Study the drawing (mm; zero at the part's minimum x, y, z) and answer. A direction names the side the tool comes from. Coordinates: 2 decimals unless noted, no trailing zeros. Write each loop counter-clockwise with the first axis right and the second up, starting at its lowest first coordinate (ties: lowest second). Pieces come first, ordered by that corner, then holes. Notation, with made-up numbers: (-16, -21) -> (27, -21) arc R15 ccw to (27, -17) -> close; hole circle Ø1 at (63.25, -21.75). An arc over 180 degrees is marked (long way). Write each question's results on one line, items separated by ' | '. Start each with the question number.
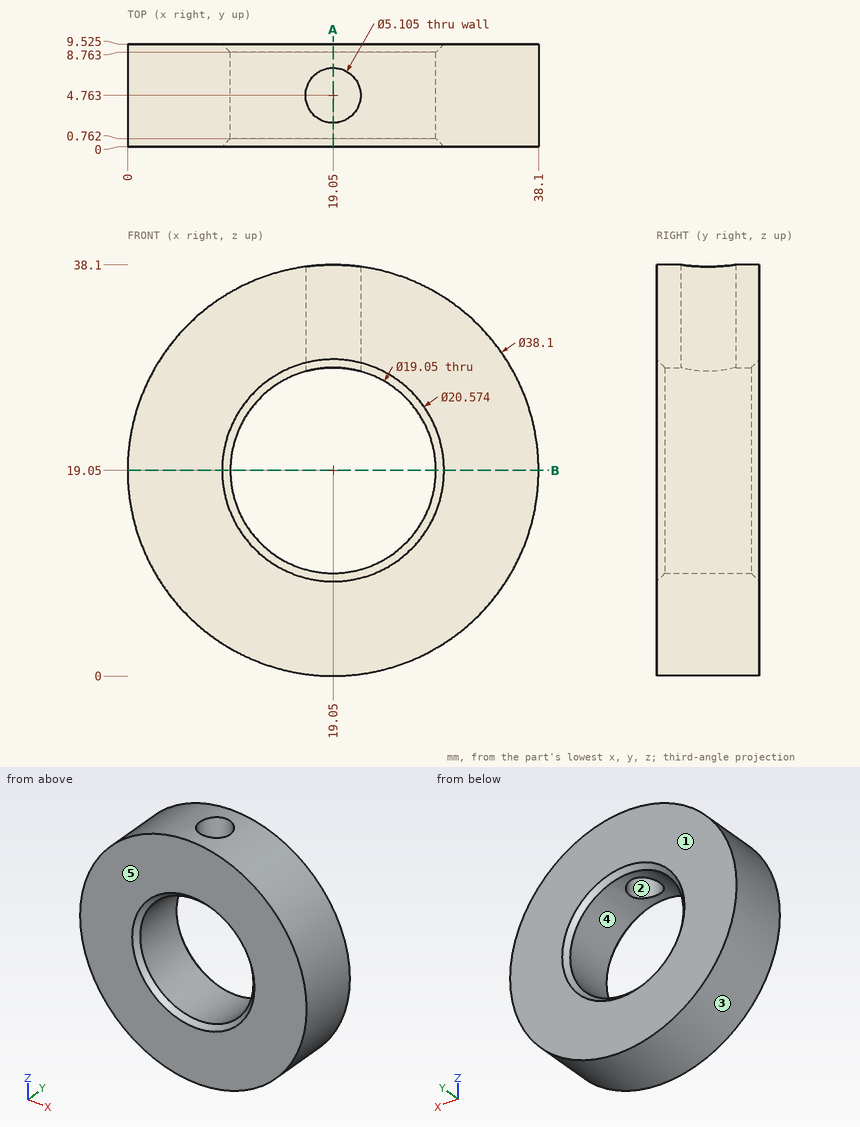
1. Find the intervals of material crossed by L1, parallel to Y at x = 19.05, z = 32 (1 decimal); L2, parallel to Z at x = 19.05, y = 4.25 (1 decimal); L3, parallel to Z at x = 24, y = 8.25 (1 decimal), in increasing order.
2. Determine the mould class of the marked faces 3, 4 and 5 for opening direction X: pulls with the +X half, pulls with the -X half, needs draft (parallel to the pull), parting line crosses it, or undercut.
3. For the marked faces 1 and 2, determine the directions among +Z, -Z, +X, -X, +Y, -Y from which every point of the face is accessible in a straight line to the end or side of a thin tool.
4. Find section B-B on z = 19.05. Give the vertices of the cut face in (x, y) (1 decimal).
5. Given pin 1 Ø1 at (x, y) = (7, 4.5) entering from +Z; pin 2 Ø3 at (x, y) = (19.05, 4.76) entering from -Z; pin 3 Ø2 at (x, y) = (5.5, 2.5) entering from -Z, each flat-ended and moving along its own axis, determine where each tip first touches the part or whether it passes through.
6. Find section A-A on x = 19.05. Give the vertices of the cut face in (y, z) (1 decimal).
Ans:
1) L1: y = 0 to 2.2, 7.3 to 9.5 | L2: z = 0 to 9.5 | L3: z = 0.7 to 10.9, 27.2 to 37.4
2) face 3: parting line crosses it | face 4: undercut | face 5: needs draft
3) face 1: +Z, -Z, +X, -X, +Y | face 2: +Z
4) outline: (0, 0) -> (8.8, 0) -> (9.5, 0.8) -> (9.5, 8.8) -> (8.8, 9.5) -> (0, 9.5) -> close; (28.6, 0.8) -> (29.3, 0) -> (38.1, 0) -> (38.1, 9.5) -> (29.3, 9.5) -> (28.6, 8.8) -> close
5) pin 1: stops at z = 34.2 | pin 2: stops at z = 0 | pin 3: stops at z = 4.72
6) outline: (0, 0) -> (9.5, 0) -> (9.5, 8.8) -> (8.8, 9.5) -> (0.8, 9.5) -> (0, 8.8) -> close; (0, 29.3) -> (0.8, 28.6) -> (2.2, 28.6) -> (2.2, 38.1) -> (0, 38.1) -> close; (7.3, 28.6) -> (8.8, 28.6) -> (9.5, 29.3) -> (9.5, 38.1) -> (7.3, 38.1) -> close
